from build123d import *

# Parameters (mm, degrees)
F0_R     = 3.25
F1_DEPTH = 3


with BuildPart() as f1:
    # F0 (on Top) → F1 (new body)
    with BuildSketch(Plane.XY):
        with BuildLine():
            Line((140.522992, -30), (221.515708, -30))
            ThreePointArc((221.515708, -30), (222.247942, -28.232233), (224.015708, -27.5))
            Line((224.015708, -27.5), (224.015708, -2.5))
            ThreePointArc((224.015708, -2.5), (221.515708, 0), (224.015708, 2.5))
            Line((224.015708, 2.5), (224.015708, 39.658693))
            Line((224.015708, 39.658693), (224.015708, 40.341307))
            ThreePointArc((224.015708, 40.341307), (215.8523, 47.998179), (208.022992, 40))
            Line((208.022992, 40), (208.022992, 15.787397))
            ThreePointArc((208.022992, 15.787397), (206.558526, 12.251863), (203.022992, 10.787397))
            Line((203.022992, 10.787397), (146.022964, 10.787397))
            ThreePointArc((146.022964, 10.787397), (142.48743, 12.251863), (141.022964, 15.787397))
            Line((141.022964, 15.787397), (141.022964, 19.978657))
            ThreePointArc((141.022964, 19.978657), (134.272065, 27.901887), (125.406482, 22.447196))
            Line((125.406482, 22.447196), (125.120118, 21.242808))
            Line((125.120118, 21.242808), (124.569344, 18.926368))
            ThreePointArc((124.569344, 18.926368), (122.326762, 15.825483), (118.54836, 15.218571))
            Line((118.54836, 15.218571), (21.81836, 38.21781))
            ThreePointArc((21.81836, 38.21781), (18.717476, 40.460392), (18.110564, 44.238793))
            Line((18.110564, 44.238793), (18.749643, 46.926629))
            Line((18.749643, 46.926629), (18.855966, 47.3738))
            ThreePointArc((18.855966, 47.3738), (11.975902, 56.943045), (3.027641, 49.272689))
            Line((3.027641, 49.272689), (0.224039, 37.481321))
            ThreePointArc((0.224039, 37.481321), (0.651558, 34.019478), (3.238437, 31.679566))
            Line((3.238437, 31.679566), (80.460392, 0.924996))
            ThreePointArc((80.460392, 0.924996), (83.707969, 2.322581), (85.105555, -0.924996))
            Line((85.105555, -0.924996), (134.872984, -20.745471))
            ThreePointArc((134.872984, -20.745471), (137.161226, -22.584387), (138.022992, -25.390633))
            Line((138.022992, -25.390633), (138.022992, -27.5))
            ThreePointArc((138.022992, -27.5), (139.790759, -28.232233), (140.522992, -30))
        make_face()
        with Locations((11.022992, 49)):
            Circle(F0_R, mode=Mode.SUBTRACT)
        with Locations((133.022992, 20)):
            Circle(F0_R, mode=Mode.SUBTRACT)
        with Locations((216.022992, 40)):
            Circle(F0_R, mode=Mode.SUBTRACT)
        with BuildLine():
            Line((206.022992, -85), (219.015708, -85))
            ThreePointArc((219.015708, -85), (222.551242, -83.535534), (224.015708, -80))
            Line((224.015708, -80), (224.015708, -32.5))
            ThreePointArc((224.015708, -32.5), (222.247942, -31.767767), (221.515708, -30))
            Line((221.515708, -30), (140.522992, -30))
            ThreePointArc((140.522992, -30), (139.790759, -31.767767), (138.022992, -32.5))
            Line((138.022992, -32.5), (138.022992, -80))
            ThreePointArc((138.022992, -80), (139.487459, -83.535534), (143.022992, -85))
            Line((143.022992, -85), (156.022992, -85))
            ThreePointArc((156.022992, -85), (159.558526, -83.535534), (161.022992, -80))
            Line((161.022992, -80), (161.022992, -50))
            ThreePointArc((161.022992, -50), (162.487459, -46.464466), (166.022992, -45))
            Line((166.022992, -45), (196.022992, -45))
            ThreePointArc((196.022992, -45), (199.558526, -46.464466), (201.022992, -50))
            Line((201.022992, -50), (201.022992, -80))
            ThreePointArc((201.022992, -80), (202.487459, -83.535534), (206.022992, -85))
        make_face()
    extrude(amount=F1_DEPTH)


solid = f1.part
Read the model definition and answer for the solid it produces. Units are mm, in the model's axes. A direction names the side the tool comes from. Give positions to 0.01 mm unless a question says otherwise; leave off trailing zeros. Loops run counter-clockwise (first coordinate to the right, second up) from the corner with the lowest first, then second, coordinate; pieces in that order, holes last. Notation, with made-up numbers: (-33, 6) - (6, 6) arc R24 ccw to (6, 28) - close; hole circle Ø8 at (31, 45.25). An arc over 180 degrees is marked (long way). Answer as CSV lines item,"result". Start each with the question number.
1) Determine the mould class of faces 1 (the face through (216, 48, 1)), 2 (the face through (222.512, -83.574, 1.479)), 3 (the face through (139.45, -83.5, 1.48)) for opening direction X: released by +X, released by -X, zero draft, split by the parting line, or undercut.
2) Find section B-B (z = 2.2). State how many separate pieces and enclosed holes the cut face has, then the cut area to 3 significant figures.
3) Which of the six approach directions +Z, -Z, +X, -X, +Y, -Y give full straight-line access (tool end or side, diameter ignored) to faces 4 (the face through (206.597, 12.291, 1.479)), 5 (the face through (153, -3, 3)), 6 (the face through (202.45, -83.5, 1.48))?
4) Each of these flat-tipped pins is pushed along its axis until it touches: pin 1 Ø1.5 at (x, z) = (174, 2) entering from +Y; pin 2 Ø0.9 at (y, z) = (-49.5, 1.5) entering from -X; pin 3 Ø5 at (x, y) = (133.02, 20) entering from -Z; pin 4 Ø1.5 at (x, z) = (183, 1) entering from -Y. Where does it stop, or does it pass through?
5) Find section A-A (y = -70.5). Write down the section's boundary in (x, z), then the cut area to 3 significant figures.
6) Straight lines are drawn through the part: L1, parallel to X at y = -50.5, z = 2.8; L2, parallel to X at y = -38.5, z = 1.75; L3, parallel to X at y = 48.5, z = 1.1. For each, find the intervals that lie inside material, in ascending order. Write a range as from..to.
7) Find section C-C (x = 185). Write down the section's boundary in (y, z).
Findings below:
1,face 1,"undercut"
1,face 2,"released by +X"
1,face 3,"released by -X"
2,separate pieces,"1"
2,enclosed holes,"3"
2,area,"10,500 mm^2"
3,face 4,"+Z, -Z, +Y"
3,face 5,"+Z, +X, -X, +Y, -Y"
3,face 6,"+Z, -Z, -Y"
4,pin 1,"y = 10.79"
4,pin 2,"x = 138.02"
4,pin 3,"through"
4,pin 4,"y = -45"
5,outline,"(138.02, 0) - (161.02, 0) - (161.02, 3) - (138.02, 3) - close; (201.02, 0) - (224.02, 0) - (224.02, 3) - (201.02, 3) - close"
5,area,"138 mm^2"
6,L1,"138.02..161.02, 201.02..224.02"
6,L2,"138.02..224.02"
6,L3,"2.84..7.81, 14.23..19.01"
7,outline,"(-45, 0) - (10.79, 0) - (10.79, 3) - (-45, 3) - close"
